Autodesk Inventor part; units mm, degrees
ref_plane "YZ Plane" through (0, 0, 0) normal (1, 0, 0) x (0, 1, 0)
ref_plane "XZ Plane" through (0, 0, 0) normal (0, 1, 0) x (-1, 0, 0)
ref_plane "XY Plane" through (0, 0, 0) normal (0, 0, 1) x (1, 0, 0)
sketch "Sketch1" plane through (0, 0, 0) normal (0, 0, 1) x (1, 0, 0)
  line L0 (0, 0) -> (1419, 0)
  line L1 (0, 330.2) -> (174.4, 330.2)
  arc A0 (174.4, 330.2) -> (182.3871, 330.3047) centre (174.4, 635) ccw
  line L2 (182.3871, 330.3047) -> (1385.6129, 361.8453)
  arc A1 (1393.6, 361.95) -> (1385.6129, 361.8453) centre (1393.6, 57.15) ccw
  line L3 (1393.6, 361.95) -> (1419, 361.95)
  line L4 (1419, 361.95) -> (1419, 412.496)
  line L5 (1419, 412.496) -> (1393.6, 412.496)
  line L6 (1393.6, 412.496) -> (1393.6, 415.925)
  line L7 (1365.025, 412.75) -> (1317.4, 412.75)
  arc A2 (1317.4, 412.75) -> (1309.4129, 412.6453) centre (1317.4, 107.95) ccw
  line L8 (1309.4129, 412.6453) -> (106.1871, 381.1047)
  arc A3 (98.2, 381) -> (106.1871, 381.1047) centre (98.2, 685.8) ccw
  line L9 (98.2, 381) -> (85.725, 381)
  line L10 (25.4, 415.925) -> (25.4, 412.496)
  line L11 (25.4, 412.496) -> (0, 412.496)
  line L12 (0, 412.496) -> (0, 330.2)
  line L13 (85.725, 381) -> (50.8, 415.925)
  line L14 (50.8, 415.925) -> (25.4, 415.925)
  line L15 (1365.025, 412.75) -> (1368.2, 415.925)
  line L16 (1368.2, 415.925) -> (1393.6, 415.925)
  dimension "d0" = 1419
  dimension "d1" = 660.4
  dimension "d2" = 723.9
  dimension "d3" = 824.992
  dimension "d4" = 50.8
  dimension "d5" = 25.4
  dimension "d6" = 25.4
  dimension "d7" = 824.992
  dimension "d8" = 762
  dimension "d9" = 25.4
  dimension "d10" = 101.6
  dimension "d11" = 304.8
  dimension "d12" = 304.8
  dimension "d13" = 1219.2
  dimension "d14" = 52.7793
  dimension "d17" = 25.4
  dimension "d18" = 45
  dimension "d19" = 831.85
  dimension "d23" = 25.4
  dimension "d24" = 45
  dimension "d25" = 831.85
revolve "Revolution1" add sketch "Sketch1" angle 360 about axis through (0, 0, 0) along (1, 0, 0)
fillet "Fillet1" radius 0.7937 2 edges at (1393.6, -412.496, 0) (25.4, -412.496, 0)
properties part number "A1-19027-200-04 HCWi reducer" material "Iron, HCWI"
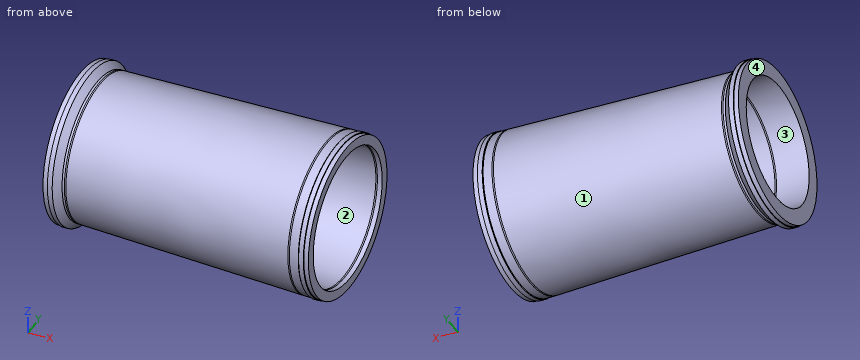
Geometry check sheet. Reference: the model listing, model coordinates, mm. Face numbers are marked on the shaded views. Coordinates: 2 decimals unless noted, no trailing zeros. Loops run counter-clockwise (first coordinate to the right, second up) from the corner with the lowest first, then second, coordinate; pieces in that order, holes last. Notation, with made-up numbers: (-3, 48.5) - (42, 48.5) arc R16 ccw to (42, 77.5) - close; hole circle Ø9 at (82.25, 85). An arc over 180 degrees is marked (long way). Use one line per item in the form item = value. Start each with the question number.
Item 1: Gauge pin test, flat ends, axial feed: pin 1 (3 mm diameter, centred on x = 907, y = -260, fed in from -Z); pin 2 (8 mm diameter, centred on x = 475, z = -283.5, fed in from +Y); pin 3 (5 mm diameter, centred on x = 1176.5, z = 0.5, fed in from +Y). Record the tip position at first contact, or that the pin passes through.
Item 2: Section check B-B, the plane x = 342. Enter the section's corners in (y, z), and give its area (3 significant figures).
Item 3: Section check A-A, the plane x = 994. Enter the section's corners in (y, z).
Item 4: Thickness scan on probe 1 along Z at (x, y) = (1409, 0); probe 2 along Z at (x, y) = (917, 325.5); probe 3 along Y at (x, z) = (676.5, -171.5). Record the ranges inside material, lowest first.
Item 5: Mould release check, pull along X, two halves, no side actions. Record for the marked faces 1, 2, 3 and 4: +X half, -X half, draft (parallel to the pull), parting line (faces both ways), or undercut.
Computed:
q1.pin_1 = -307.99
q1.pin_2 = 273.1
q1.pin_3 = 409.23
q2.outline = circle Ø774.57 at (0, 0); hole circle Ø668.98 at (0, 0)
q2.area = 120,000 mm2
q3.outline = circle Ø808.75 at (0, 0); hole circle Ø703.16 at (0, 0)
q4.probe_1 = -412.5 to -361.95, 361.95 to 412.5
q4.probe_2 = -236.52 to -127.45, 127.45 to 236.52
q4.probe_3 = -357 to -297.34, 297.34 to 357
q5.face_1 = undercut
q5.face_2 = +X half
q5.face_3 = draft
q5.face_4 = -X half
